Input: part model. Units: mm. Frame: model coordinates. Round coordinates to 2 decimals unless told otherwise and drop trailing zeros. Loops run counter-clockwise (first coordinate to the right, second up) from the corner with the lowest first, then second, coordinate; pieces in that order, holes last. Notation, with made-up numbers: (55.25, -32.5) - (82.25, -32.5) arc R24 ccw to (82.25, 2.5) - close; hole circle Ø3 at (83, 14). An arc over 180 degrees is marked (long way). Write each question's results on one line, items separated by ' | '.
from build123d import *

# Parameters (mm, degrees)
SKETCH1_R           = 9.525
BOSS_EXTRUDE1_DEPTH = 406.4
SKETCH3_R           = 12.7
BOSS_EXTRUDE2_DEPTH = 12.7


with BuildPart() as part:
    # Sketch1 → Boss-Extrude1 (new body)
    with BuildSketch(Plane(origin=(0, 0, 0), x_dir=(0, 0, -1), z_dir=(1, 0, 0))):
        Circle(SKETCH1_R)
    extrude(amount=BOSS_EXTRUDE1_DEPTH)

    # Sketch2 → Revolve1 (revolve)
    with BuildSketch(Plane.XY, mode=Mode.PRIVATE) as revolve1_sk:
        with BuildLine():
            Line((-9.525, 0), (0, 0))
            Line((0, 0), (0, 9.525))
            ThreePointArc((0, 9.525), (-6.735192091, 6.735192091), (-9.525, 0))
        make_face()
    revolve(revolve1_sk.sketch.rotate(Axis((-9.525, 0, 0), (1, 0, 0)), 90), axis=Axis((-9.525, 0, 0), (1, 0, 0)))

    # Sketch3 → Boss-Extrude2 (add)
    with BuildSketch(Plane(origin=(406.4, 0, 0), x_dir=(0, 0, -1), z_dir=(1, 0, 0))):
        Circle(SKETCH3_R)
    extrude(amount=BOSS_EXTRUDE2_DEPTH)


solid = part.part
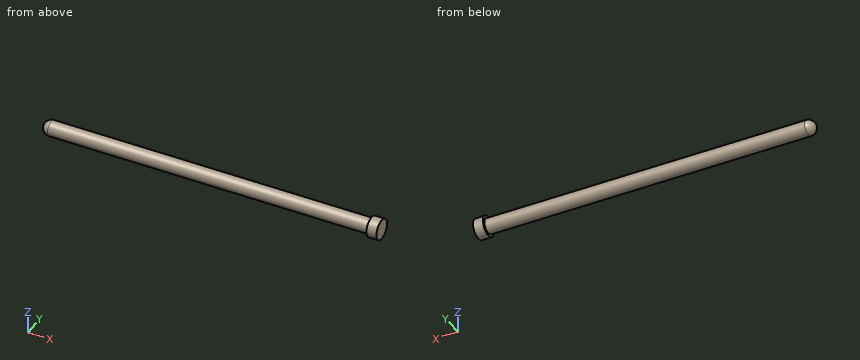
1. Section query A-A, the plane z = 0. Output: boundary loops of the cut face in (x, y) (3 decimals), plus the area to 3 significant figures.
Answer:
outline: (0, -9.525) - (406.4, -9.525) - (406.4, -12.7) - (419.1, -12.7) - (419.1, 12.7) - (406.4, 12.7) - (406.4, 9.525) - (0, 9.525) arc R9.525 ccw to start | area: 8,210 mm^2
2. Line query: line 1 (X direction, y = 3.25, z = -11.25); line 2 (Z direction, x = 244, y = -1); line 3 (Y direction, x = 275.5, z = 0.25). Output: solid intervals per line, ascending. Write a range as [from, to].
Answer:
line 1: [406.4, 419.1] | line 2: [-9.47, 9.47] | line 3: [-9.52, 9.52]
3. Contact query for flat-ended pins moving along their axis: pin 1 (1 mm diameter, centred on x = 359.5, z = 6, fed in from +Y); pin 2 (10 mm diameter, centred on x = 186.5, z = 5, fed in from -Y) (3 decimals); pin 3 (3 mm diameter, centred on y = 9, z = 6.5, fed in from -X). Output: stop coordinate, or through.
Answer:
pin 1: y = 7.78 | pin 2: y = -9.525 | pin 3: x = 406.4
4. Section query B-B, the plane y = 4.75. Output: boundary loops of the cut face in (x, z), plus the area to 3 significant figures.
Answer:
outline: (0, -8.26) - (406.4, -8.26) - (406.4, -11.78) - (419.1, -11.78) - (419.1, 11.78) - (406.4, 11.78) - (406.4, 8.26) - (0, 8.26) arc R8.26 ccw to start | area: 7,120 mm^2
5. Section query C-C, the plane x = 49. Output: boundary loops of the cut face in (y, z) (3 decimals), plus the area to 3 significant figures.
Answer:
outline: circle Ø19.05 at (0, 0) | area: 285 mm^2
